from build123d import *
from OCP.BRepFilletAPI import BRepFilletAPI_MakeChamfer

# Parameters (mm, degrees)
SKETCH1_W           = 84
SKETCH1_H           = 66
BOSS_EXTRUDE1_DEPTH = 3
CHAMFER2_SIZE       = 6
CHAMFER4_SIZE       = 3
CHAMFER4_SIZE_2     = 6
SKETCH2_R           = 1.75
CUT_EXTRUDE1_DEPTH  = 54.4976635


with BuildPart() as part:
    # Sketch1 → Boss-Extrude1 (new body)
    with BuildSketch(Plane.XY):
        Rectangle(SKETCH1_W, SKETCH1_H)
    extrude(amount=BOSS_EXTRUDE1_DEPTH)

    # Chamfer2
    chamfer2_edges = [part.edges().sort_by_distance(p)[0] for p in [
        (42, -33, 1.5),
        (-42, -33, 1.5),
        (-42, 33, 1.5),
        (42, 33, 1.5),
    ]]
    chamfer(chamfer2_edges, length=CHAMFER2_SIZE)

    # Chamfer4
    chamfer4_edges_1 = [part.edges().sort_by_distance(p)[0] for p in [
        (0, -33, 3),
    ]]
    chamfer4_side_1 = [part.faces().sort_by_distance(p)[0] for p in [
        (0, -33, 2.94),
    ]]
    chamfer4_edges_2 = [part.edges().sort_by_distance(p)[0] for p in [
        (0, 33, 3),
    ]]
    chamfer4_side_2 = [part.faces().sort_by_distance(p)[0] for p in [
        (0, 32.94, 3),
    ]]
    chamfer4 = BRepFilletAPI_MakeChamfer(part.part.solid().wrapped)
    for e in chamfer4_edges_1:
        chamfer4.Add(CHAMFER4_SIZE - 0.0001, CHAMFER4_SIZE_2 - 0.0001, e.wrapped, chamfer4_side_1[0].wrapped)
    for e in chamfer4_edges_2:
        chamfer4.Add(CHAMFER4_SIZE_2 - 0.0001, CHAMFER4_SIZE - 0.0001, e.wrapped, chamfer4_side_2[0].wrapped)
    add(Compound.cast(chamfer4.Shape()), mode=Mode.REPLACE)  # a hair under: the kernel refuses the full size

    # Sketch2 → Cut-Extrude1 (cut, through all)
    with BuildSketch(Plane.XY.offset(3)):
        with Locations((-39, -19)):
            Circle(SKETCH2_R)
        with Locations(Location((39, -19, 0), (0, 0, 180))):
            Circle(SKETCH2_R)
        with Locations((39, 16)):
            Circle(SKETCH2_R)
        with Locations(Location((-39, 16, 0), (0, 0, 180))):
            Circle(SKETCH2_R)
    extrude(amount=-CUT_EXTRUDE1_DEPTH, mode=Mode.SUBTRACT)


solid = part.part
Geometry: final body of the model. Coordinates: model frame, mm. Give positions to 0.01 mm unless a question says otherwise; leave off trailing zeros. Order: outer loops, then holes, each group sorted by start corner. A loop starts at its lowest first (then second) coordinate and runs counter-clockwise, first axis right, second up. Notation, with made-up numbers: (10, 7.25) -> (46, 7.25) arc R23 ccw to (46, 42.25) -> close; hole circle Ø1 at (15.25, 68.5). An arc over 180 degrees is marked (long way). Put each result on its own line as item: value.
Q1. Section D-D, the plane y = 28.5. Return loops of the section in (x, z), then the cut area to 3 significant figures.
Here are the results:
outline: (-40.5, 0) -> (40.5, 0) -> (40.5, 2.25) -> (-40.5, 2.25) -> close
area: 182 mm^2
Q2. Material intervals for L1, parallel to Y at x = -39, z = 2.2; L2, parallel to X at y = 16.5, z = 2.4; L3, parallel to Y at x = -39, z = 2.1, sorted ascending.
Here are the results:
L1: y = -28.6 to -20.75, -17.25 to 14.25, 17.75 to 28.6
L2: x = -42 to -40.68, -37.32 to 37.32, 40.68 to 42
L3: y = -28.8 to -20.75, -17.25 to 14.25, 17.75 to 28.8
Q3. Draft query along X for faces 1 (the face through (-42, 0, 1)), 2 (the face through (-38.1, -17.5, 1.5)), 3 (the face through (40, 29, 1)). Return one class per face: released by +X, released by -X, zero draft, split by the parting line, or undercut.
Here are the results:
face 1: released by -X
face 2: undercut
face 3: released by +X
Q4. Section B-B, the plane z = 2. Return loops of the section in (x, y), then the cut area to 3 significant figures.
Here are the results:
outline: (-42, -27) -> (-40, -29) -> (40, -29) -> (42, -27) -> (42, 27) -> (40, 29) -> (-40, 29) -> (-42, 27) -> close; hole circle Ø3.5 at (-39, -19); hole circle Ø3.5 at (-39, 16); hole circle Ø3.5 at (39, -19); hole circle Ø3.5 at (39, 16)
area: 4,830 mm^2
Q5. Section A-A, the plane y = -19. Return loops of the section in (x, z), then the cut area to 3 significant figures.
Here are the results:
outline: (-42, 0) -> (-40.75, 0) -> (-40.75, 3) -> (-42, 3) -> close; (-37.25, 0) -> (37.25, 0) -> (37.25, 3) -> (-37.25, 3) -> close; (40.75, 0) -> (42, 0) -> (42, 3) -> (40.75, 3) -> close
area: 231 mm^2
Q6. Section C-C, the plane x = 39. Return loops of the section in (y, z), then the cut area to 4 significant figures.
Here are the results:
outline: (-30, 0) -> (-20.75, 0) -> (-20.75, 3) -> (-27, 3) -> (-30, 1.5) -> close; (-17.25, 0) -> (14.25, 0) -> (14.25, 3) -> (-17.25, 3) -> close; (17.75, 0) -> (30, 0) -> (30, 1.5) -> (27, 3) -> (17.75, 3) -> close
area: 154.5 mm^2
